Can you work these out from the model? Positions are in its coordinate system, mm. A direction names the side the tool comes from. Give positions to 0.01 mm unless a question says otherwise; leave off trailing zeros. Order: outer loops, then holes, each group sorted by start corner. A loop starts at its lowest first (then second) coordinate and runs counter-clockwise, first axis right, second up. Notation, with made-up numbers: (61, 57.25) - (96, 57.25) arc R23 cw to (96, 81.25) - close; hole circle Ø11 at (-3, 37). An arc over 180 degrees is marked (long way). Use one line per item in the form item = value. Start each with the question number.
1) Suppose I cut it at B-B, the plane x = 4. Write out the boundary of the cut face in (y, z).
2) Suppose I cut it at D-D, the plane z = 15. Write out the boundary of the cut face in (x, y).
3) Which directions (+Z, -Z, +X, -X, +Y, -Y) give clear straight access to the entire face, cutting with the end or side of a thin tool? Please do faces 4 (the flat face through (0, 15, 12)), 5 (the cylindrical face through (-0.99, 5.13, 13.77)).
4) We'd pull the mould along Y, two halves only. Please class faces 1 (the cylindrical face through (2.722, -0.986, 2.334)), 2 (the cylindrical face through (-0.986, 22.003, 12.631)), 3 (the flat face through (-1, 24, 12)): released by +Y, released by -Y, zero draft, split by the parting line, or undercut.
5) Please list where these lines run through material, in increasing order: probe 1 along X at (y, z) = (-0.65, 20); probe 2 along Z at (x, y) = (-1.5, 4); probe 3 along Y at (x, z) = (0.5, 15.5).
6) Suppose I cut it at A-A, the plane z = 12. State how many separate pieces and enclosed holes the cut face has, and give its area (3 significant figures).
7) For pin 1 (6.5 mm diameter, centred on y = 4, z = 12, fed in from +X); pin 2 (2.5 mm diameter, centred on x = 12, z = 4, fed in from -Y); pin 3 (1.5 mm diameter, centred on x = 11, z = 21, fed in from +Y), each with a flat end and sliding along its axis, tell me the tip position at first contact or that it passes through.
```python
from build123d import *

# Parameters (mm, degrees)
EXTRU_MINCE1_DEPTH              = 24
ESQUISSE2_R                     = 2.1
ENL_V_MAT_EXTRU_1_DEPTH         = 42.569219382
R_P_TITION_LIN_AIRE1_COUNT      = 3
R_P_TITION_LIN_AIRE1_PITCH      = 8
R_P_TITION_LIN_AIRE1_COUNT_DIR2 = 3
R_P_TITION_LIN_AIRE1_PITCH_DIR2 = 8
ESQUISSE3_R                     = 2.1
ENL_V_MAT_EXTRU_2_DEPTH         = 42.569219382
R_P_TITION_LIN_AIRE2_COUNT      = 3
R_P_TITION_LIN_AIRE2_PITCH      = 8
R_P_TITION_LIN_AIRE2_COUNT_DIR2 = 3
R_P_TITION_LIN_AIRE2_PITCH_DIR2 = 8


with BuildPart() as part:
    # Esquisse1 → Extru.-Mince1 (new body)
    with BuildSketch(Plane.XY):
        Polygon((0, 24), (0, 0), (24, 0), (24, -2), (-2, -2), (-2, 24), align=None)
    extrude(amount=EXTRU_MINCE1_DEPTH)

    # Esquisse2 → Enlèv. mat.-Extru.1 (cut, through all)
    with BuildSketch(Plane(origin=(0, 0, 0), x_dir=(1, 0, 0), z_dir=(0, 1, 0))):
        with Locations(Location((4, -20, 0), (0, 0, 270))):
            Circle(ESQUISSE2_R)
    enl_v_mat_extru_1 = extrude(amount=-ENL_V_MAT_EXTRU_1_DEPTH, mode=Mode.SUBTRACT)

    # Répétition linéaire1: Enl_v. mat.-Extru.1 3 × 3
    with Locations(*[(i * R_P_TITION_LIN_AIRE1_PITCH, 0, -j * R_P_TITION_LIN_AIRE1_PITCH_DIR2) for i in range(R_P_TITION_LIN_AIRE1_COUNT) for j in range(R_P_TITION_LIN_AIRE1_COUNT_DIR2) if (i, j) != (0, 0)]):
        add(enl_v_mat_extru_1, mode=Mode.SUBTRACT)

    # Esquisse3 → Enlèv. mat.-Extru.2 (cut, through all)
    with BuildSketch(Plane(origin=(0, 0, 0), x_dir=(0, 0, -1), z_dir=(1, 0, 0))):
        with Locations(Location((-20, 4, 0), (0, 0, 90))):
            Circle(ESQUISSE3_R)
    enl_v_mat_extru_2 = extrude(amount=-ENL_V_MAT_EXTRU_2_DEPTH, mode=Mode.SUBTRACT)

    # Répétition linéaire2: Enl_v. mat.-Extru.2 3 × 3
    with Locations(*[(0, i * R_P_TITION_LIN_AIRE2_PITCH, -j * R_P_TITION_LIN_AIRE2_PITCH_DIR2) for i in range(R_P_TITION_LIN_AIRE2_COUNT) for j in range(R_P_TITION_LIN_AIRE2_COUNT_DIR2) if (i, j) != (0, 0)]):
        add(enl_v_mat_extru_2, mode=Mode.SUBTRACT)


solid = part.part
```
Result sheet:
q1.outline = (-2, 0) - (0, 0) - (0, 1.9) - (-2, 1.9) - close; (-2, 6.1) - (0, 6.1) - (0, 9.9) - (-2, 9.9) - close; (-2, 14.1) - (0, 14.1) - (0, 17.9) - (-2, 17.9) - close; (-2, 22.1) - (0, 22.1) - (0, 24) - (-2, 24) - close
q2.outline = (-2, -2) - (24, -2) - (24, 0) - (0, 0) - (0, 24) - (-2, 24) - close
q3.face_4 = +Z, -Z, +X, +Y
q3.face_5 = +X, -X
q4.face_1 = zero draft
q4.face_2 = undercut
q4.face_3 = released by +Y
q5.probe_1 = -2 to 1.9, 6.1 to 9.9, 14.1 to 17.9, 22.1 to 24
q5.probe_2 = 0 to 1.9, 6.1 to 9.9, 14.1 to 17.9, 22.1 to 24
q5.probe_3 = -2 to 0
q6.separate_pieces = 7
q6.enclosed_holes = 0
q6.area = 49.6 mm²
q7.pin_1 = 0
q7.pin_2 = through
q7.pin_3 = 0
